```python
from build123d import *

# Parameters (mm, degrees)
SKETCH021_W             = 51.5
SKETCH021_H             = 3
PAD014_DEPTH            = 1.6
SKETCH022_R             = 3
PAD015_DEPTH            = 2.6
HOLE_D                  = 3.4
HOLE_DEPTH              = 25
HOLE_CSINK_D            = 6.7
HOLE_CSINK_ANGLE        = 90
BODY005_PLACEMENT_ANGLE = 180


with BuildPart() as part:
    # Sketch021 → Pad014 (new body)
    with BuildSketch(Plane.XY):
        with BuildLine():
            ThreePointArc((-54, 40), (-57.535534, 38.535534), (-59, 35))
            Line((-59, -35), (-59, 35))
            ThreePointArc((-59, -35), (-57.535534, -38.535534), (-54, -40))
            Line((54, -40), (-54, -40))
            ThreePointArc((54, -40), (57.535534, -38.535534), (59, -35))
            Line((59, 35), (59, -35))
            ThreePointArc((59, 35), (57.535534, 38.535534), (54, 40))
            Line((-54, 40), (54, 40))
        make_face()
        with Locations((0, 21.5)):
            Rectangle(SKETCH021_W, SKETCH021_H, mode=Mode.SUBTRACT)
        with Locations((0, -21.5)):
            Rectangle(SKETCH021_W, SKETCH021_H, mode=Mode.SUBTRACT)
    extrude(amount=PAD014_DEPTH)

    # Sketch022 → Pad015 (join)
    with BuildSketch(Plane.XY):
        with Locations((-55, 36)):
            Circle(SKETCH022_R)
        with Locations((1, 36)):
            Circle(SKETCH022_R)
        with Locations((55, 36)):
            Circle(SKETCH022_R)
        with Locations((55, -36)):
            Circle(SKETCH022_R)
        with Locations((1, -36)):
            Circle(SKETCH022_R)
        with Locations((-55, -36)):
            Circle(SKETCH022_R)
    extrude(amount=PAD015_DEPTH)

    # Hole
    with Locations(Plane(origin=(0, 0, 0), x_dir=(1, 0, 0), z_dir=(0, 0, -1))):
        with Locations((-55, -36), (1, -36), (55, -36), (55, 36), (1, 36), (-55, 36)):
            CounterSinkHole(HOLE_D / 2, HOLE_CSINK_D / 2, depth=HOLE_DEPTH, counter_sink_angle=HOLE_CSINK_ANGLE)


with BuildPart() as part_1:
    # Body005 placement: moved
    add(part.part.moved(Location((0, 0, 100))).rotate(Axis((0, 0, 100), (1, 0, 0)), BODY005_PLACEMENT_ANGLE))


solid = part_1.part
```
Source: CAD feature listing. Evaluate the final solid. Frame: model axes, mm. A direction names the side the tool comes from. Coordinates: 2 decimals unless noted, no trailing zeros. Loops run counter-clockwise (first coordinate to the right, second up) from the corner with the lowest first, then second, coordinate; pieces in that order, holes last. Notation, with made-up numbers: M 49.5,-21.5 L 55.5,-21.5 A22 ccw 55.5,11.5 Z; hole C -4,80 d2. An arc over 180 degrees is marked long. Put each result on its own line as item: value. Start each with the question number.
1) Pull-direction query (X, two-part tool) for faces 1 (the face through (1.37, 34.34, 97.87)), 2 (the face through (-57, -39, 99)), 3 (the face through (55, 38, 97.4)); classes: pulls with the +X half, pulls with the -X half, needs draft (parallel to the pull), parting line crosses it, or undercut.
2) Reachability of faces 4 (the face through (52.79, -38.03, 97.91)), 5 (the face through (-53.65, 34.97, 97.87)) from +Z, -Z, +X, -X, +Y, -Y: full face, straight path, thin tool, end or side. Return the list, or none.
3) Cut plane D-D on x = 29. Return the cut outline in (y, z).
4) Contact query for flat-ended pins moving along their axis: pin 1 Ø24 at (x, y) = (-21.5, 12) entering from -Z; pin 2 Ø1.5 at (x, z) = (45.5, 98) entering from +Y; pin 3 Ø4.5 at (x, y) = (55, 36) entering from +Z. Output: stop coordinate, or through.
5) Cut plane A-A on x = -21.5. Return the cut outline in (y, z).
6) Cut plane B-B on z = 98.9. Give the number of separate pieces and of enclosed holes in the cut face, then the cut area to 3 significant figures.
7) Cut plane C-C on y = -7. Return the cut outline in (x, z).
8) Ray query, L1, parallel to X at y = -36, z = 97.8; L2, parallel to Y at x = -10, z = 99.75; L3, parallel to Y at x = 55, z = 98.1. Return the intervals inside material, ascending. Write a range as from..to.
The answers:
1. face 1: undercut
1. face 2: pulls with the -X half
1. face 3: needs draft
2. face 4: -Z
2. face 5: +Z, -Z
3. outline: M -40,98.4 L 40,98.4 L 40,100 L -40,100 Z
4. pin 1: stops at z = 98.4
4. pin 2: stops at y = 40
4. pin 3: stops at z = 98.9
5. outline: M -40,98.4 L -23,98.4 L -23,100 L -40,100 Z; M -20,98.4 L 20,98.4 L 20,100 L -20,100 Z; M 23,98.4 L 40,98.4 L 40,100 L 23,100 Z
6. separate pieces: 1
6. enclosed holes: 8
6. area: 9,010 mm²
7. outline: M -59,98.4 L 59,98.4 L 59,100 L -59,100 Z
8. L1: x = -58..-56.7, -53.3..-52, -2..-0.7, 2.7..4, 52..53.3, 56.7..58
8. L2: y = -40..-23, -20..20, 23..40
8. L3: y = -39..-37.7, -34.3..-33, 33..34.3, 37.7..39
